Part model, mm, in its own coordinate system. Face numbers are marked on the shaded views. A direction names the side the tool comes from. Give positions to 0.01 mm unless a question says otherwise; leave off trailing zeros. Write each loop counter-clockwise with the first axis right and the second up, starting at its lowest first coordinate (ties: lowest second). Pieces come first, ordered by that corner, then holes.
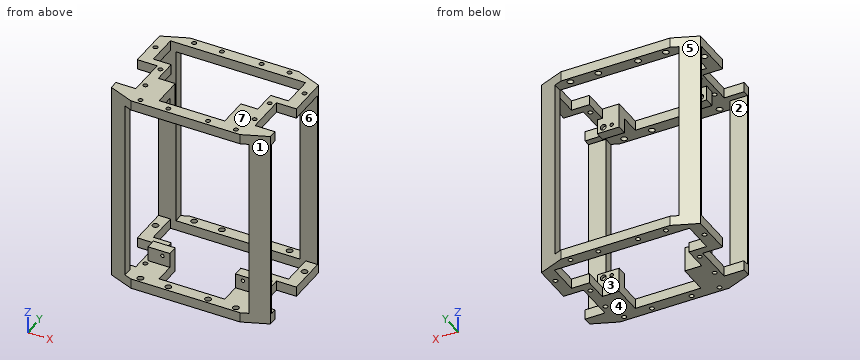
from build123d import *

# Parameters (mm, degrees)
SKETCH1_R                 = 2.25
BOSS_EXTRUDE2_DEPTH       = 202.6
SKETCH2_W                 = 182.6
SKETCH2_H                 = 86
CUT_EXTRUDE1_DEPTH        = 161
SKETCH4_R                 = 3
CUT_EXTRUDE2_DEPTH        = 4.5
CUT_EXTRUDE3_START        = 182.6
SKETCH4_2_R               = 3
CUT_EXTRUDE3_DEPTH        = 4.5
SKETCH3_W                 = 110
SKETCH3_H                 = 182.6
CUT_EXTRUDE4_DEPTH        = 111
CUT_EXTRUDE5_START        = -12
SKETCH5_W                 = 125
SKETCH5_H                 = 182.6
CUT_EXTRUDE5_DEPTH        = 111
SKETCH6_W                 = 20
SKETCH6_H                 = 40
CUT_EXTRUDE7_DEPTH        = 12
SKETCH8_R                 = 2.25
BOSS_EXTRUDE3_DEPTH       = 10
BOSS_EXTRUDE4_START       = -192.6
SKETCH8_2_R               = 2.25
BOSS_EXTRUDE4_DEPTH       = 10
BOSS_EXTRUDE5_START       = 30
SKETCH9_W                 = 2
SKETCH9_H                 = 10
SKETCH9_W_2               = 15
SKETCH9_H_2               = 5
SKETCH9_R                 = 1.75
BOSS_EXTRUDE5_DEPTH       = 10
SKETCH10_W                = 22
SKETCH10_H                = 10
BOSS_EXTRUDE6_DEPTH       = 20
MIRROR3_START             = 30
MIRROR3_COPY_1_SKETCH_W   = 2
MIRROR3_COPY_1_SKETCH_H   = 10
MIRROR3_COPY_1_SKETCH_W_2 = 15
MIRROR3_COPY_1_SKETCH_H_2 = 5
MIRROR3_COPY_1_SKETCH_R   = 1.75
MIRROR3_COPY_1_DEPTH      = 10
MIRROR3_COPY_2_SKETCH_W   = 22
MIRROR3_COPY_2_SKETCH_H   = 10
MIRROR3_COPY_2_DEPTH      = 20
SKETCH11_R                = 2.25
CUT_EXTRUDE8_DEPTH        = 203.6
SKETCH12_R                = 3
CUT_EXTRUDE9_DEPTH        = 3.1


with BuildPart() as part:
    # Sketch1 → Boss-Extrude2 (new body)
    with BuildSketch(Plane.XY):
        Polygon((-48.624838984, -50.035732152), (61.375161016, -50.035732152), (86.375161016, -40.035732152), (86.375161016, 49.964267848), (61.375161016, 59.964267848), (-48.624838984, 59.964267848), (-73.624838984, 49.964267848), (-73.624838984, -40.035732152), align=None)
        with Locations((-41.624838984, -45.035732152)):
            Circle(SKETCH1_R, mode=Mode.SUBTRACT)
        with Locations((-68.624838984, -23.035732152)):
            Circle(SKETCH1_R, mode=Mode.SUBTRACT)
        with Locations((-13.624838984, -45.035732152)):
            Circle(SKETCH1_R, mode=Mode.SUBTRACT)
        with Locations((-68.624838984, 4.964267848)):
            Circle(SKETCH1_R, mode=Mode.SUBTRACT)
        with Locations((26.375161016, -45.035732152)):
            Circle(SKETCH1_R, mode=Mode.SUBTRACT)
        with Locations((54.375161016, -45.035732152)):
            Circle(SKETCH1_R, mode=Mode.SUBTRACT)
        with Locations((81.375161016, -23.035732152)):
            Circle(SKETCH1_R, mode=Mode.SUBTRACT)
        Polygon((74.375161016, 47.964267848), (74.375161016, -38.035732152), (13.375161016, -38.035732152), (-0.624838984, -38.035732152), (-61.624838984, -38.035732152), (-61.624838984, 47.964267848), (-7.624838984, 47.964267848), (-0.624838984, 47.964267848), (13.375161016, 47.964267848), (20.375161016, 47.964267848), align=None, mode=Mode.SUBTRACT)
        with Locations((81.375161016, 4.964267848)):
            Circle(SKETCH1_R, mode=Mode.SUBTRACT)
        with Locations((-68.624838984, 32.964267848)):
            Circle(SKETCH1_R, mode=Mode.SUBTRACT)
        with Locations((-41.624838984, 54.964267848)):
            Circle(SKETCH1_R, mode=Mode.SUBTRACT)
        with Locations((-13.624838984, 54.964267848)):
            Circle(SKETCH1_R, mode=Mode.SUBTRACT)
        with Locations((26.375161016, 54.964267848)):
            Circle(SKETCH1_R, mode=Mode.SUBTRACT)
        with Locations((81.375161016, 32.964267848)):
            Circle(SKETCH1_R, mode=Mode.SUBTRACT)
        with Locations((54.375161016, 54.964267848)):
            Circle(SKETCH1_R, mode=Mode.SUBTRACT)
    extrude(amount=BOSS_EXTRUDE2_DEPTH)

    # Sketch2 → Cut-Extrude1 (cut, through all)
    with BuildSketch(Plane.ZY.offset(73.624838984)):
        with Locations((101.3, 4.964267848)):
            Rectangle(SKETCH2_W, SKETCH2_H)
    extrude(amount=-CUT_EXTRUDE1_DEPTH, mode=Mode.SUBTRACT)

    # Sketch4 → Cut-Extrude2 (cut)
    with BuildSketch(Plane.XY.offset(10)):
        with Locations((-68.624838984, 32.964267848)):
            Circle(SKETCH4_R)
        with Locations((-68.624838984, 4.964267848)):
            Circle(SKETCH4_R)
        with Locations((-68.624838984, -23.035732152)):
            Circle(SKETCH4_R)
        with Locations((-41.624838984, 54.964267848)):
            Circle(SKETCH4_R)
        with Locations((-13.624838984, 54.964267848)):
            Circle(SKETCH4_R)
        with Locations((26.375161016, 54.964267848)):
            Circle(SKETCH4_R)
        with Locations((54.375161016, 54.964267848)):
            Circle(SKETCH4_R)
        with Locations((81.375161016, 32.964267848)):
            Circle(SKETCH4_R)
        with Locations((81.375161016, 4.964267848)):
            Circle(SKETCH4_R)
        with Locations((81.375161016, -23.035732152)):
            Circle(SKETCH4_R)
        with Locations((54.375161016, -45.035732152)):
            Circle(SKETCH4_R)
        with Locations((26.375161016, -45.035732152)):
            Circle(SKETCH4_R)
        with Locations((-13.624838984, -45.035732152)):
            Circle(SKETCH4_R)
        with Locations((-41.624838984, -45.035732152)):
            Circle(SKETCH4_R)
    extrude(amount=-CUT_EXTRUDE2_DEPTH, mode=Mode.SUBTRACT)

    # Sketch4<2> → Cut-Extrude3 (cut)
    with BuildSketch(Plane.XY.offset(10).offset(CUT_EXTRUDE3_START)):
        with Locations((-68.624838984, 32.964267848)):
            Circle(SKETCH4_2_R)
        with Locations((-68.624838984, 4.964267848)):
            Circle(SKETCH4_2_R)
        with Locations((-68.624838984, -23.035732152)):
            Circle(SKETCH4_2_R)
        with Locations((-41.624838984, 54.964267848)):
            Circle(SKETCH4_2_R)
        with Locations((-13.624838984, 54.964267848)):
            Circle(SKETCH4_2_R)
        with Locations((26.375161016, 54.964267848)):
            Circle(SKETCH4_2_R)
        with Locations((54.375161016, 54.964267848)):
            Circle(SKETCH4_2_R)
        with Locations((81.375161016, 32.964267848)):
            Circle(SKETCH4_2_R)
        with Locations((81.375161016, 4.964267848)):
            Circle(SKETCH4_2_R)
        with Locations((81.375161016, -23.035732152)):
            Circle(SKETCH4_2_R)
        with Locations((54.375161016, -45.035732152)):
            Circle(SKETCH4_2_R)
        with Locations((26.375161016, -45.035732152)):
            Circle(SKETCH4_2_R)
        with Locations((-13.624838984, -45.035732152)):
            Circle(SKETCH4_2_R)
        with Locations((-41.624838984, -45.035732152)):
            Circle(SKETCH4_2_R)
    extrude(amount=CUT_EXTRUDE3_DEPTH, mode=Mode.SUBTRACT)

    # Sketch3 → Cut-Extrude4 (cut, through all)
    with BuildSketch(Plane(origin=(0, 59.964267848, 0), x_dir=(1, 0, 0), z_dir=(0, 1, 0))):
        with Locations((6.375161016, -101.3)):
            Rectangle(SKETCH3_W, SKETCH3_H)
    extrude(amount=-CUT_EXTRUDE4_DEPTH, mode=Mode.SUBTRACT)

    # Sketch5 → Cut-Extrude5 (cut, through all)
    with BuildSketch(Plane(origin=(0, -38.035732152, 0), x_dir=(1, 0, 0), z_dir=(0, 1, 0)).offset(CUT_EXTRUDE5_START)):
        with Locations((6.375161016, -101.3)):
            Rectangle(SKETCH5_W, SKETCH5_H)
    extrude(amount=CUT_EXTRUDE5_DEPTH, mode=Mode.SUBTRACT)

    # Sketch6 → Cut-Extrude7 (cut)
    with BuildSketch(Plane(origin=(86.375161016, 0, 0), x_dir=(0, 0, -1), z_dir=(1, 0, 0))):
        with Locations((-192.6, -11.535732152)):
            Rectangle(SKETCH6_W, SKETCH6_H)
        with Locations((-10, -11.535732152)):
            Rectangle(SKETCH6_W, SKETCH6_H)
    cut_extrude7 = extrude(amount=-CUT_EXTRUDE7_DEPTH, mode=Mode.SUBTRACT)

    # Sketch8 → Boss-Extrude3 (add)
    with BuildSketch(Plane.XY.offset(202.6)):
        Polygon((66.375161016, 8.464267848), (66.375161016, -31.535732152), (74.375161016, -31.535732152), (74.375161016, -38.035732152), (56.375161016, -38.035732152), (56.375161016, 15.998735889), (74.375161016, 15.998735889), (74.375161016, 8.464267848), align=None)
        with Locations((61.375161016, 4.964267848)):
            Circle(SKETCH8_R, mode=Mode.SUBTRACT)
        with Locations((61.375161016, -23.035732152)):
            Circle(SKETCH8_R, mode=Mode.SUBTRACT)
    boss_extrude3 = extrude(amount=-BOSS_EXTRUDE3_DEPTH)

    # Sketch8<2> → Boss-Extrude4 (add)
    with BuildSketch(Plane.XY.offset(202.6).offset(BOSS_EXTRUDE4_START)):
        Polygon((66.375161016, 8.464267848), (66.375161016, -31.535732152), (74.375161016, -31.535732152), (74.375161016, -38.035732152), (56.375161016, -38.035732152), (56.375161016, 15.998735889), (74.375161016, 15.998735889), (74.375161016, 8.464267848), align=None)
        with Locations((61.375161016, 4.964267848)):
            Circle(SKETCH8_2_R, mode=Mode.SUBTRACT)
        with Locations((61.375161016, -23.035732152)):
            Circle(SKETCH8_2_R, mode=Mode.SUBTRACT)
    boss_extrude4 = extrude(amount=-BOSS_EXTRUDE4_DEPTH)

    # Mirror1: Cut-Extrude7, Boss-Extrude3, Boss-Extrude4 across plane
    add(cut_extrude7.mirror(Plane(origin=(6.375161016, 0, 0), x_dir=(0, 0, 1), z_dir=(1, 0, 0))), mode=Mode.SUBTRACT)
    add(boss_extrude3.mirror(Plane(origin=(6.375161016, 0, 0), x_dir=(0, 0, 1), z_dir=(1, 0, 0))))
    add(boss_extrude4.mirror(Plane(origin=(6.375161016, 0, 0), x_dir=(0, 0, 1), z_dir=(1, 0, 0))))

    # Sketch9 → Boss-Extrude5 (add)
    with BuildSketch(Plane(origin=(0, -38.035732152, 0), x_dir=(1, 0, 0), z_dir=(0, 1, 0)).offset(BOSS_EXTRUDE5_START)):
        Polygon((-48.624838984, -25), (-41.624838984, -25), (-41.624838984, -15), (-41.624838984, -10), (-43.624838984, -10), (-43.624838984, 0), (-48.624838984, 0), align=None)
        with Locations((-42.624838984, -5)):
            Rectangle(SKETCH9_W, SKETCH9_H)
        with Locations((-34.124838984, -5)):
            Rectangle(SKETCH9_W_2, SKETCH9_H)
        with Locations((-34.124838984, -12.5)):
            Rectangle(SKETCH9_W_2, SKETCH9_H_2)
        with Locations((-34.124838984, -20)):
            Rectangle(SKETCH9_W_2, SKETCH9_H)
        with Locations((-34.124838984, -20)):
            Circle(SKETCH9_R, mode=Mode.SUBTRACT)
    boss_extrude5 = extrude(amount=-BOSS_EXTRUDE5_DEPTH)

    # Sketch10 → Boss-Extrude6 (add)
    with BuildSketch(Plane.XZ.offset(18.035732152)):
        with Locations((-37.624838984, 5)):
            Rectangle(SKETCH10_W, SKETCH10_H)
    boss_extrude6 = extrude(amount=BOSS_EXTRUDE6_DEPTH)

    # Mirror2: Boss-Extrude5, Boss-Extrude6 across plane
    add(boss_extrude5.mirror(Plane.XY.offset(101.3)))
    add(boss_extrude6.mirror(Plane.XY.offset(101.3)))

    # Mirror3: Boss-Extrude5, Boss-Extrude6 across plane
    add(boss_extrude5.mirror(Plane(origin=(6.375161016, 0, 0), x_dir=(0, 0, 1), z_dir=(1, 0, 0))))
    add(boss_extrude6.mirror(Plane(origin=(6.375161016, 0, 0), x_dir=(0, 0, 1), z_dir=(1, 0, 0))))

    # Mirror3 copy 1 sketch → Mirror3 copy 1 (add)
    with BuildSketch(Plane(origin=(12.750322031, -38.035732152, 202.6), x_dir=(-1, 0, 0), z_dir=(0, 1, 0)).offset(MIRROR3_START)):
        Polygon((-48.624838984, -25), (-41.624838984, -25), (-41.624838984, -15), (-41.624838984, -10), (-43.624838984, -10), (-43.624838984, 0), (-48.624838984, 0), align=None)
        with Locations((-42.624838984, -5)):
            Rectangle(MIRROR3_COPY_1_SKETCH_W, MIRROR3_COPY_1_SKETCH_H)
        with Locations((-34.124838984, -5)):
            Rectangle(MIRROR3_COPY_1_SKETCH_W_2, MIRROR3_COPY_1_SKETCH_H)
        with Locations((-34.124838984, -12.5)):
            Rectangle(MIRROR3_COPY_1_SKETCH_W_2, MIRROR3_COPY_1_SKETCH_H_2)
        with Locations((-34.124838984, -20)):
            Rectangle(MIRROR3_COPY_1_SKETCH_W_2, MIRROR3_COPY_1_SKETCH_H)
        with Locations((-34.124838984, -20)):
            Circle(MIRROR3_COPY_1_SKETCH_R, mode=Mode.SUBTRACT)
    extrude(amount=-MIRROR3_COPY_1_DEPTH)

    # Mirror3 copy 2 sketch → Mirror3 copy 2 (add)
    with BuildSketch(Plane(origin=(12.750322031, -18.035732152, 202.6), x_dir=(-1, 0, 0), z_dir=(0, -1, 0))):
        with Locations((-37.624838984, 5)):
            Rectangle(MIRROR3_COPY_2_SKETCH_W, MIRROR3_COPY_2_SKETCH_H)
    extrude(amount=MIRROR3_COPY_2_DEPTH)

    # Sketch11 → Cut-Extrude8 (cut, through all)
    with BuildSketch(Plane.XY.offset(202.6)):
        with Locations((-48.624838984, -23.035732152)):
            Circle(SKETCH11_R)
        with Locations((61.375161016, -23.035732152)):
            Circle(SKETCH11_R)
    extrude(amount=-CUT_EXTRUDE8_DEPTH, mode=Mode.SUBTRACT)

    # Sketch12 → Cut-Extrude9 (cut)
    with BuildSketch(Plane(origin=(0, -8.035732152, 0), x_dir=(1, 0, 0), z_dir=(0, 1, 0))):
        with Locations((-42.624838984, -20)):
            Circle(SKETCH12_R)
        with Locations((55.375161016, -20)):
            Circle(SKETCH12_R)
        with Locations((55.375161016, -182.6)):
            Circle(SKETCH12_R)
        with Locations((-42.624838984, -182.6)):
            Circle(SKETCH12_R)
    extrude(amount=-CUT_EXTRUDE9_DEPTH, mode=Mode.SUBTRACT)


solid = part.part
1) Mould opens along Z. For the marked faces 4, 5, 6 and 7 say: +Z half, -Z half, draft (parallel to the pull), parting line (faces both ways), or undercut.
Check result:
face 4: -Z half
face 5: draft
face 6: undercut
face 7: +Z half
2) Saw through at B-B (z = 65.5). Write the cut outline in (x, y).
Check result:
outline: (-73.62, -40.04) - (-56.12, -47.04) - (-56.12, -38.04) - (-73.62, -38.04) - close; (-73.62, 47.96) - (-56.12, 47.96) - (-56.12, 56.96) - (-73.62, 49.96) - close; (68.88, -47.04) - (86.38, -40.04) - (86.38, -38.04) - (68.88, -38.04) - close; (68.88, 47.96) - (86.38, 47.96) - (86.38, 49.96) - (68.88, 56.96) - close
3) Saw through at A-A (y = -2.5). Write the cut outline in (x, z).
Check result:
outline: (-53.62, 0) - (-43.62, 0) - (-43.62, 10) - (-53.62, 10) - close; (-53.62, 192.6) - (-43.62, 192.6) - (-43.62, 202.6) - (-53.62, 202.6) - close; (56.38, 0) - (66.38, 0) - (66.38, 10) - (56.38, 10) - close; (56.38, 192.6) - (66.38, 192.6) - (66.38, 202.6) - (56.38, 202.6) - close
4) Drill centre lines: L1, parallel to X at y = -9.4, z = 182.6; L2, parallel to Z at x = -49.5, y = -4; L3, parallel to Y at x = 52.5, z = 14.5. Where is each one in solid material? Low to high.
Check result:
L1: x = -48.62 to -45.62, -39.62 to -35.87, -32.37 to -26.62, 39.38 to 45.13, 48.63 to 52.38, 58.38 to 61.38
L2: z = 0 to 10, 192.6 to 202.6
L3: y = -18.04 to -8.04
5) 3-axis set-ups, long thin cutter, end or side, ignore diameter. For the marked faces 1, 2 and 3: which of +Z, -Z, +X, -X, +Y, -Y reach the whole face in a straight line?
Check result:
face 1: +Z, -Z, +X, -Y
face 2: +X, -X
face 3: none
6) Saw through at C-C (x = 71.5). Write the cut outline in (y, z), and give its area (3 significant figures).
Check result:
outline: (-45.99, 0) - (-31.54, 0) - (-31.54, 10) - (-38.04, 10) - (-38.04, 192.6) - (-31.54, 192.6) - (-31.54, 202.6) - (-45.99, 202.6) - close; (8.46, 0) - (16, 0) - (16, 10) - (8.46, 10) - close; (8.46, 192.6) - (16, 192.6) - (16, 202.6) - (8.46, 202.6) - close; (47.96, 0) - (55.91, 0) - (55.91, 202.6) - (47.96, 202.6) - close
area: 3,500 mm2
7) Flat gauge pins, fed straight in: P1, Ø1, axis at x = 36, y = 46, coming from the -Z side; P2, Ø8, axis at x = -59.5, z = 196, coming from the -Y side; P3, Ø5, axis at x = 77.5, z = 3, coming from the +Y side; P4, Ø3, axis at y = -7.5, z = 197, coming from the +X side. Where does each tip first touch, or does it go through?
Check result:
P1: passes through
P2: stops at y = -47.29
P3: stops at y = 54.51
P4: stops at x = 66.38
